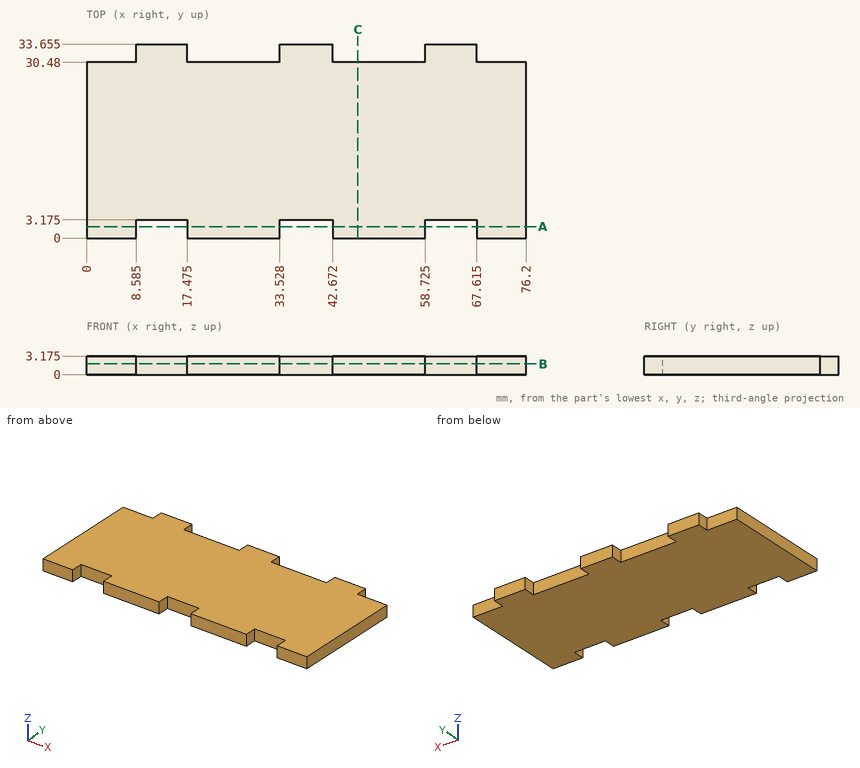
Check sheet for the drawn part. Datum: minimum x, y, z corner. Units: mm. Coordinates: 2 decimals unless noted, no trailing zeros. Loops run counter-clockwise (first coordinate to the right, second up) from the corner with the lowest first, then second, coordinate; pieces in that order, holes last. Notation, with made-up numbers: (36, -2.5) - (46, -2.5) arc R28 cw to (46, 26.5) - close; hole circle Ø1 at (-9, -38). An arc over 180 degrees is marked (long way). Put each result on its own line as item: value.
Item 1: Section check C-C (x = 47). Enter the section's corners in (y, z) (3 decimals).
Conclusion:
outline: (0, 0) - (30.48, 0) - (30.48, 3.175) - (0, 3.175) - close
Item 2: Scan lines: line 1 along X through (y, z) = (2, 2.9) (1 decimal); line 2 along X through (y, z) = (31, 2.8) (1 decimal); line 3 along Y through (x, z) = (63.5, 2.25) (3 decimals). Record each from-to range of solid material in increasing order.
Conclusion:
line 1: x = 0 to 8.6, 17.5 to 33.5, 42.7 to 58.7, 67.6 to 76.2
line 2: x = 8.6 to 17.5, 33.5 to 42.7, 58.7 to 67.6
line 3: y = 3.175 to 33.655
Item 3: Section check A-A (y = 2). Enter the section's corners in (x, z) (1 decimal).
Conclusion:
outline: (0, 0) - (8.6, 0) - (8.6, 3.2) - (0, 3.2) - close; (17.5, 0) - (33.5, 0) - (33.5, 3.2) - (17.5, 3.2) - close; (42.7, 0) - (58.7, 0) - (58.7, 3.2) - (42.7, 3.2) - close; (67.6, 0) - (76.2, 0) - (76.2, 3.2) - (67.6, 3.2) - close
Item 4: Gauge pin test, flat end, axial feed: pin 1 Ø1.6 at (y, z) = (31.5, 2) entering from +X (3 decimals). Record the tip position at first contact, or that the pin passes through.
Conclusion:
pin 1: stops at x = 67.615
Item 5: Section check B-B (z = 1.85). Enter the section's corners in (x, y) (1 decimal).
Conclusion:
outline: (0, 0) - (8.6, 0) - (8.6, 3.2) - (17.5, 3.2) - (17.5, 0) - (33.5, 0) - (33.5, 3.2) - (42.7, 3.2) - (42.7, 0) - (58.7, 0) - (58.7, 3.2) - (67.6, 3.2) - (67.6, 0) - (76.2, 0) - (76.2, 30.5) - (67.6, 30.5) - (67.6, 33.7) - (58.7, 33.7) - (58.7, 30.5) - (42.7, 30.5) - (42.7, 33.7) - (33.5, 33.7) - (33.5, 30.5) - (17.5, 30.5) - (17.5, 33.7) - (8.6, 33.7) - (8.6, 30.5) - (0, 30.5) - close
